Design review of the part built by this model. Coordinates are the model's own, in mm. A direction names the side the tool comes from. Coordinates: 2 decimals unless noted, no trailing zeros. Loops run counter-clockwise (first coordinate to the right, second up) from the corner with the lowest first, then second, coordinate; pieces in that order, holes last. Notation, with made-up numbers: M 75.25,74 L 103.25,74 A32 cw 103.25,104 Z; hole C -21,-23.5 d4. An arc over 180 degrees is marked long. Put each result on its own line as item: value. Start each with the question number.
(1) Take a section at D-D, the plane z = 1. Give the boundary of the cut face in (x, y) (3 decimals).
(2) For probe 1 along Y at (x, z) = (-7, -1.5); probe 2 along X at (y, z) = (-4, 11); probe 3 along Z at (x, y) = (-15.5, -6.25), list the stretches that pass through material, from the lowest coordinate up. Write a range as [from, to].
(3) The part is to be moulded in two halves that separate along Z. For faces 4 (the flat face through (2, -4, -15.875)), 5 (the flat face through (10, -4, -1.651)), 6 (the flat face through (-15.875, -4, -2)), 7 (the flat face through (-14, -4, 3.759)), say which applies: +Z half, -Z half, draft (parallel to the pull), parting line (faces both ways), or undercut.
(4) Clearance check with flat-ended pins moving along their axes: pin 1 (1.5 mm diameter, centred on y = -3.5, z = -6.5, fed in from -X); pin 2 (2.5 mm diameter, centred on y = -2, z = -0.5, fed in from -X) (3 decimals); pin 3 (2.5 mm diameter, centred on x = 0, y = -4.5, fed in from +Z) (3 decimals). State where each tip first meets the part, or that it passes through.
(5) Take a section at A-A, the plane y = -1.5. Give the boundary of the cut face in (x, z) (3 decimals), then the cut area to 3 significant figures.
(6) Take a section at B-B, the plane z = 10.5. Give the boundary of the cut face in (x, y), then the cut area to 3 significant figures.
(7) For faces 1 (the flat face through (-10, -5.41, 0)), 2 (the flat face through (3.759, -4, 14)), 3 (the flat face through (15.875, -4, 2)), list the 3-axis set-ups (+Z, -Z, +X, -X, +Y, -Y) from which the entire face can be reached by the end or side of a thin tool; tool diameter is ignored.
(8) Take a section at C-C, the plane x = 7.5. Give the boundary of the cut face in (y, z), then the cut area to 3 significant figures.
```python
from build123d import *

# Parameters (mm, degrees)
BOSS_EXTRUDE1_DEPTH = 7.5184
SKETCH2_W           = 3.302
SKETCH2_H           = 3.302
CUT_EXTRUDE1_DEPTH  = 12.7
CIRPATTERN1_COUNT   = 4
BOSS_EXTRUDE2_DEPTH = 2.54


with BuildPart() as part:
    # Sketch1 → Boss-Extrude1 (new body)
    with BuildSketch(Plane(origin=(0, 0, 0), x_dir=(1, 0, 0), z_dir=(0, 1, 0))):
        with BuildLine():
            Line((3.7592, 11.3792), (3.7592, 15.875))
            Line((3.7592, 15.875), (-3.7592, 15.875))
            Line((-3.7592, 15.875), (-3.7592, 11.3792))
            ThreePointArc((-3.7592, 11.3792), (-5.991046327, 5.991046327), (-11.3792, 3.7592))
            Line((-11.3792, 3.7592), (-15.875, 3.7592))
            Line((-15.875, 3.7592), (-15.875, -3.7592))
            Line((-15.875, -3.7592), (-11.3792, -3.7592))
            ThreePointArc((-11.3792, -3.7592), (-5.991046327, -5.991046327), (-3.7592, -11.3792))
            Line((-3.7592, -11.3792), (-3.7592, -15.875))
            Line((-3.7592, -15.875), (3.7592, -15.875))
            Line((3.7592, -15.875), (3.7592, -11.3792))
            ThreePointArc((3.7592, -11.3792), (5.991046327, -5.991046327), (11.3792, -3.7592))
            Line((11.3792, -3.7592), (15.875, -3.7592))
            Line((15.875, -3.7592), (15.875, 3.7592))
            Line((15.875, 3.7592), (11.3792, 3.7592))
            ThreePointArc((11.3792, 3.7592), (5.991046327, 5.991046327), (3.7592, 11.3792))
        make_face()
    extrude(amount=-BOSS_EXTRUDE1_DEPTH)

    # Sketch2 → Cut-Extrude1 (cut)
    with BuildSketch(Plane.XY.offset(15.875)):
        with Locations((0, -3.7592)):
            Rectangle(SKETCH2_W, SKETCH2_H)
    cut_extrude1 = extrude(amount=-CUT_EXTRUDE1_DEPTH, mode=Mode.SUBTRACT)

    # CirPattern1: Cut-Extrude1 ×4 about axis
    cirpattern1_axis = Axis((0, 0, 0), (0, 1, 0))
    for i in range(1, CIRPATTERN1_COUNT):
        add(cut_extrude1.rotate(cirpattern1_axis, i * 360 / CIRPATTERN1_COUNT), mode=Mode.SUBTRACT)

    # Sketch4 → Boss-Extrude2 (add)
    with BuildSketch(Plane(origin=(0, 0, 0), x_dir=(1, 0, 0), z_dir=(0, 1, 0))):
        Polygon((3.7592, 19.05), (19.05, 3.7592), (19.05, -3.7592), (3.7592, -19.05), (-3.7592, -19.05), (-19.05, -3.7592), (-19.05, 3.7592), (-3.7592, 19.05), align=None)
    extrude(amount=BOSS_EXTRUDE2_DEPTH)


solid = part.part
```
Computed values:
1. outline: M -19.05,0 L -15.875,0 L -15.875,-2.108 L -3.175,-2.108 L -3.175,-5.41 L -15.875,-5.41 L -15.875,-7.518 L 15.875,-7.518 L 15.875,-5.41 L 3.175,-5.41 L 3.175,-2.108 L 15.875,-2.108 L 15.875,0 L 19.05,0 L 19.05,2.54 L -19.05,2.54 Z
2. probe 1: y = [-7.52, -5.41], [-2.11, 2.54]
2. probe 2: x = [-3.77, -1.65], [1.65, 3.77]
2. probe 3: z = [-3.76, 3.76]
3. face 4: -Z half
3. face 5: undercut
3. face 6: draft
3. face 7: +Z half
4. pin 1: stops at x = -6.24
4. pin 2: stops at x = -15.875
4. pin 3: stops at z = 15.875
5. outline: M -15.875,-3.759 L -11.379,-3.759 A7.62 cw -3.759,-11.379 L -3.759,-15.875 L 3.759,-15.875 L 3.759,-11.379 A7.62 cw 11.379,-3.759 L 15.875,-3.759 L 15.875,3.759 L 11.379,3.759 A7.62 cw 3.759,11.379 L 3.759,15.875 L -3.759,15.875 L -3.759,11.379 A7.62 cw -11.379,3.759 L -15.875,3.759 Z
5. area: 471 mm^2
6. outline: M -12.31,0 L -3.81,0 L -3.81,-7.52 L 3.81,-7.52 L 3.81,0 L 12.31,0 L 12.31,2.54 L -12.31,2.54 Z; hole M -1.65,-5.41 L 1.65,-5.41 L 1.65,-2.11 L -1.65,-2.11 Z
6. area: 109 mm^2
7. face 1: -X
7. face 2: +Z, +X, -Y
7. face 3: +Z, -Z, +X, -Y
8. outline: M -7.52,-4.82 L 0,-4.82 L 0,-15.31 L 2.54,-15.31 L 2.54,15.31 L 0,15.31 L 0,4.82 L -7.52,4.82 Z; hole M -5.41,-1.65 L -2.11,-1.65 L -2.11,1.65 L -5.41,1.65 Z
8. area: 139 mm^2
